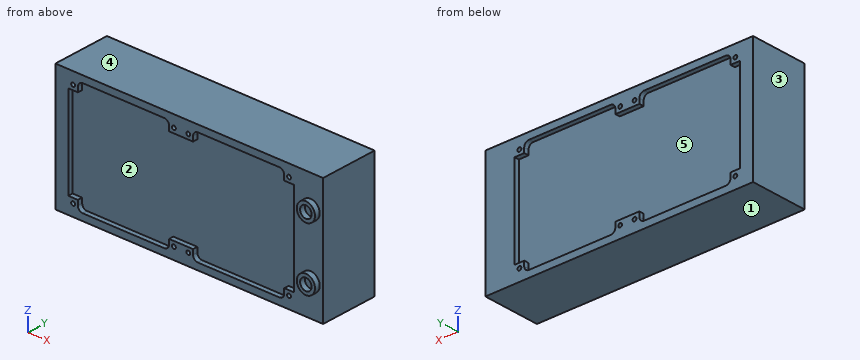
```python
from build123d import *

# Parameters (mm, degrees)
F0_W     = 279
F0_H     = 129
F1_DEPTH = 60
F2_R     = 9.5
F2_R_2   = 6
F3_DEPTH = 5.5
F4_R     = 2
F5_DEPTH = 5
F6_R     = 2
F7_DEPTH = 5


with BuildPart() as f1:
    # F0 (on Front) → F1 (new body)
    with BuildSketch(Plane.XZ):
        with Locations((139.5, 0)):
            Rectangle(F0_W, F0_H)
    extrude(amount=F1_DEPTH)

    # F2 (on face) → F3 (join)
    with BuildSketch(Plane.XZ.offset(60)):
        with Locations((266, -32)):
            Circle(F2_R)
        with Locations((266, -32)):
            Circle(F2_R_2, mode=Mode.SUBTRACT)
        with Locations((266, 32)):
            Circle(F2_R)
        with Locations((266, 32)):
            Circle(F2_R_2, mode=Mode.SUBTRACT)
    extrude(amount=F3_DEPTH)

    # F4 (on face) → F5 (cut)
    with BuildSketch(Plane.XZ.offset(60)):
        with Locations((18.5, 52.5)):
            Circle(F4_R)
        with Locations((123.5, 52.5)):
            Circle(F4_R)
        with Locations((138.5, 52.5)):
            Circle(F4_R)
        with Locations((243.5, 52.5)):
            Circle(F4_R)
        with BuildLine():
            Line((23.5, 47.5), (13.5, 47.5))
            Line((13.5, 47.5), (13.5, 0))
            Line((13.5, 0), (13.5, -47.5))
            Line((13.5, -47.5), (23.5, -47.5))
            Line((23.5, -47.5), (23.5, -52.5))
            ThreePointArc((23.5, -52.5), (24.964466, -56.035534), (28.5, -57.5))
            Line((28.5, -57.5), (113.5, -57.5))
            ThreePointArc((113.5, -57.5), (117.035534, -56.035534), (118.5, -52.5))
            Line((118.5, -52.5), (118.5, -47.5))
            Line((118.5, -47.5), (143.5, -47.5))
            Line((143.5, -47.5), (143.5, -52.5))
            ThreePointArc((143.5, -52.5), (144.964466, -56.035534), (148.5, -57.5))
            Line((148.5, -57.5), (233.5, -57.5))
            ThreePointArc((233.5, -57.5), (237.035534, -56.035534), (238.5, -52.5))
            Line((238.5, -52.5), (238.5, -47.5))
            Line((238.5, -47.5), (248.5, -47.5))
            Line((248.5, -47.5), (248.5, 0))
            Line((248.5, 0), (248.5, 47.5))
            Line((248.5, 47.5), (238.5, 47.5))
            Line((238.5, 47.5), (238.5, 52.5))
            ThreePointArc((238.5, 52.5), (237.035534, 56.035534), (233.5, 57.5))
            Line((233.5, 57.5), (148.5, 57.5))
            ThreePointArc((148.5, 57.5), (144.964466, 56.035534), (143.5, 52.5))
            Line((143.5, 52.5), (143.5, 47.5))
            Line((143.5, 47.5), (118.5, 47.5))
            Line((118.5, 47.5), (118.5, 52.5))
            ThreePointArc((118.5, 52.5), (117.035534, 56.035534), (113.5, 57.5))
            Line((113.5, 57.5), (28.5, 57.5))
            ThreePointArc((28.5, 57.5), (24.964466, 56.035534), (23.5, 52.5))
            Line((23.5, 52.5), (23.5, 47.5))
        make_face()
        with Locations((243.5, -52.5)):
            Circle(F4_R)
        with Locations((138.5, -52.5)):
            Circle(F4_R)
        with Locations((123.5, -52.5)):
            Circle(F4_R)
        with Locations((18.5, -52.5)):
            Circle(F4_R)
    extrude(amount=-F5_DEPTH, mode=Mode.SUBTRACT)

    # F6 (on face) → F7 (cut)
    with BuildSketch(Plane(origin=(0, 0, 0), x_dir=(-1, 0, 0), z_dir=(0, 1, 0))):
        with Locations((-243.5, 52.5)):
            Circle(F6_R)
        with Locations((-138.5, 52.5)):
            Circle(F6_R)
        with Locations((-123.5, 52.5)):
            Circle(F6_R)
        with Locations((-18.5, 52.5)):
            Circle(F6_R)
        with BuildLine():
            Line((-238.5, 47.5), (-248.5, 47.5))
            Line((-248.5, 47.5), (-248.5, 0))
            Line((-248.5, 0), (-248.5, -47.5))
            Line((-248.5, -47.5), (-238.5, -47.5))
            Line((-238.5, -47.5), (-238.5, -52.5))
            ThreePointArc((-238.5, -52.5), (-237.035534, -56.035534), (-233.5, -57.5))
            Line((-233.5, -57.5), (-148.5, -57.5))
            ThreePointArc((-148.5, -57.5), (-144.964466, -56.035534), (-143.5, -52.5))
            Line((-143.5, -52.5), (-143.5, -47.5))
            Line((-143.5, -47.5), (-118.5, -47.5))
            Line((-118.5, -47.5), (-118.5, -52.5))
            ThreePointArc((-118.5, -52.5), (-117.035534, -56.035534), (-113.5, -57.5))
            Line((-113.5, -57.5), (-28.5, -57.5))
            ThreePointArc((-28.5, -57.5), (-24.964466, -56.035534), (-23.5, -52.5))
            Line((-23.5, -52.5), (-23.5, -47.5))
            Line((-23.5, -47.5), (-13.5, -47.5))
            Line((-13.5, -47.5), (-13.5, 0))
            Line((-13.5, 0), (-13.5, 47.5))
            Line((-13.5, 47.5), (-23.5, 47.5))
            Line((-23.5, 47.5), (-23.5, 52.5))
            ThreePointArc((-23.5, 52.5), (-24.964466, 56.035534), (-28.5, 57.5))
            Line((-28.5, 57.5), (-113.5, 57.5))
            ThreePointArc((-113.5, 57.5), (-117.035534, 56.035534), (-118.5, 52.5))
            Line((-118.5, 52.5), (-118.5, 47.5))
            Line((-118.5, 47.5), (-143.5, 47.5))
            Line((-143.5, 47.5), (-143.5, 52.5))
            ThreePointArc((-143.5, 52.5), (-144.964466, 56.035534), (-148.5, 57.5))
            Line((-148.5, 57.5), (-233.5, 57.5))
            ThreePointArc((-233.5, 57.5), (-237.035534, 56.035534), (-238.5, 52.5))
            Line((-238.5, 52.5), (-238.5, 47.5))
        make_face()
        with Locations((-18.5, -52.5)):
            Circle(F6_R)
        with Locations((-123.5, -52.5)):
            Circle(F6_R)
        with Locations((-138.5, -52.5)):
            Circle(F6_R)
        with Locations((-243.5, -52.5)):
            Circle(F6_R)
    extrude(amount=-F7_DEPTH, mode=Mode.SUBTRACT)


solid = f1.part
```
Read the model definition and answer for the solid it produces. Units are mm, in the model's axes. Face numbers are marked on the shaded views. A direction names the side the tool comes from. Give positions to 0.01 mm unless a question says otherwise; leave off trailing zeros. Order: outer loops, then holes, each group sorted by start corner. A loop starts at its lowest first (then second) coordinate and runs counter-clockwise, first axis right, second up. Notation, with made-up numbers: (-4, -19) -> (7, -19) arc R22 cw to (7, 8) -> close; hole circle Ø2 at (16.25, 74). An arc over 180 degrees is marked (long way). One line per item, written item: value. Start each with the question number.
(1) The part is cut by section B-B (z = -6). Determine the outline of the cut face in (x, y).
(2) The part is cut by section C-C (z = 32). Determine the outline of the cut face in (x, y), and give its area (3 significant figures).
(3) The part is cut by section A-A (x = 266). Determine the outline of the cut face in (y, z).
(4) The part is cut by section D-D (x = 34). Determine the outline of the cut face in (y, z), and give its area (3 significant figures).
(5) A tool of negligible diameter and unlimited length cuts with its end or side. For the marked faces 1 and 2, from which of +Z, -Z, +X, -X, +Y, -Y can it reach the whole face along a straight path? Write none if from no direction.
(6) Flat-ended cylindrical pins translate along their axes: P1, Ø4, axis at x = 89.5, z = -22, coming from the -Y side; P2, Ø6.5, axis at x = 123.5, z = -52.5, coming from the -Y side; P3, Ø10, axis at x = 214.5, z = -46, coming from the +Y side. Find the tip coordinate at first contact, or state that the pin passes through.
(7) Straight lines are drawn through the part: L1, parallel to Z at x = 266, y = -62.1; L2, parallel to Z at x = 123, y = -3; L3, parallel to X at y = -58.5, z = 27.5. For each, find the intervals that lie inside material, in ascending order.
(8) For a pull along Z with two mould halves and no side action, classify the marked faces 3, 4 and 5 as released by +Z, released by -Z, zero draft, split by the parting line, or undercut.
Taken from the geometry:
1. outline: (0, -60) -> (13.5, -60) -> (13.5, -55) -> (248.5, -55) -> (248.5, -60) -> (279, -60) -> (279, 0) -> (248.5, 0) -> (248.5, -5) -> (13.5, -5) -> (13.5, 0) -> (0, 0) -> close
2. outline: (0, -60) -> (13.5, -60) -> (13.5, -55) -> (248.5, -55) -> (248.5, -60) -> (256.5, -60) -> (256.5, -65.5) -> (260, -65.5) -> (260, -60) -> (272, -60) -> (272, -65.5) -> (275.5, -65.5) -> (275.5, -60) -> (279, -60) -> (279, 0) -> (248.5, 0) -> (248.5, -5) -> (13.5, -5) -> (13.5, 0) -> (0, 0) -> close
2. area: 14,400 mm^2
3. outline: (-65.5, -41.5) -> (-60, -41.5) -> (-60, -64.5) -> (0, -64.5) -> (0, 64.5) -> (-60, 64.5) -> (-60, 41.5) -> (-65.5, 41.5) -> (-65.5, 38) -> (-60, 38) -> (-60, 26) -> (-65.5, 26) -> (-65.5, 22.5) -> (-60, 22.5) -> (-60, -22.5) -> (-65.5, -22.5) -> (-65.5, -26) -> (-60, -26) -> (-60, -38) -> (-65.5, -38) -> close
4. outline: (-60, -64.5) -> (0, -64.5) -> (0, -57.5) -> (-5, -57.5) -> (-5, 57.5) -> (0, 57.5) -> (0, 64.5) -> (-60, 64.5) -> (-60, 57.5) -> (-55, 57.5) -> (-55, -57.5) -> (-60, -57.5) -> close
4. area: 6,590 mm^2
5. face 1: -Z, +X, -X, +Y, -Y
5. face 2: -Y
6. P1: y = -55
6. P2: y = -60
6. P3: y = -5
7. L1: -41.5 to -38, -26 to -22.5, 22.5 to 26, 38 to 41.5
7. L2: -64.5 to -54.44, -50.56 to -47.5, 47.5 to 50.56, 54.44 to 64.5
7. L3: 0 to 13.5, 248.5 to 279
8. face 3: zero draft
8. face 4: released by +Z
8. face 5: undercut
